Input: part model. Units: mm. Frame: model coordinates. Face numbers are marked on the shaded views. Coordinates: 2 decimals unless noted, no trailing zeros. Write each loop counter-clockwise with the first axis right and the second up, starting at its lowest first coordinate (ties: lowest second). Pieces come first, ordered by that corner, then holes. Notation, with made-up numbers: (65.5, -39) - (91.5, -39) arc R32 cw to (91.5, -3) - close; hole circle Ø3 at (18, 39). An arc over 180 degrees is marked (long way). Put each result on its own line as item: value. Start each with the question number.
1. Cut plane D-D, the plane y = 2. Return loops of the section in (x, z), and give its area (3 significant figures).
2. Pull-direction query (Z, two-part tool) for the marked faces 1, 2 and 3; classes: released by +Z, released by -Z, zero draft, split by the parting line, or undercut.
3. Cut plane B-B, the plane y = -2.5. Return loops of the section in (x, z), and give its area (3 significant figures).
4. Cut plane C-C, the plane z = 0. Return loops of the section in (x, y), and give its area (3 significant figures).
5. Cut plane A-A, the plane x = 4.5. Return loops of the section in (y, z) (3 decimals).
6. Line query: line 1 (Y direction, x = 11.25, z = 0); line 2 (Y direction, x = 4.5, z = 11.5); line 3 (Y direction, x = 2.5, z = 0.5). Output: solid intervals per line, ascending.
7. Pin query (flat end, axial travel): pin 1 (2 mm diameter, centred on y = -9, z = 2.5, fed in from -X); pin 2 (8 mm diameter, centred on x = 6.5, z = -6.5, fed in from -Y); pin 3 (3 mm diameter, centred on x = 4.5, y = -6, fed in from -Z); pin 4 (1 mm diameter, centred on x = 10, z = -0.5, fed in from +Y). Return the tip coordinate at first contact, or that it passes through.
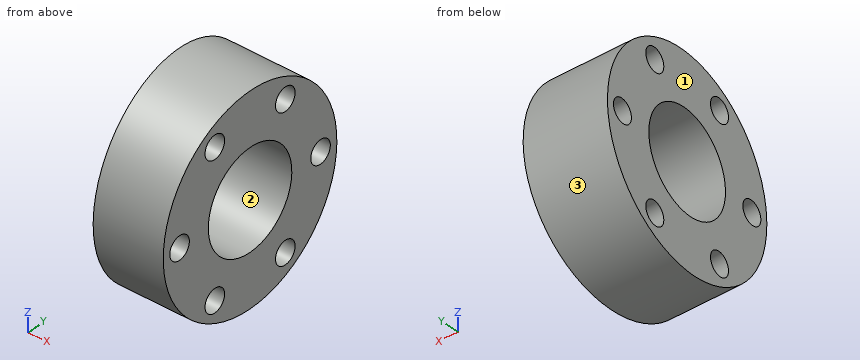
from build123d import *

# Parameters (mm, degrees)
SKETCH1_R               = 16.891
BOSS_EXTRUDE1_DEPTH     = 13.97
SKETCH2_R               = 8.128
CUT_EXTRUDE1_DEPTH      = 28.672597674
CUT_EXTRUDE2_DEPTH      = 28.672597674
CUT_EXTRUDE2_DEPTH_BACK = 28.672597674
SKETCH7_R               = 1.905
CUT_EXTRUDE3_DEPTH      = 28.672597674
CIRPATTERN1_COUNT       = 6


with BuildPart() as part:
    # Sketch1 → Boss-Extrude1 (new body)
    with BuildSketch(Plane(origin=(0, 0, 0), x_dir=(0, 0, -1), z_dir=(1, 0, 0))):
        Circle(SKETCH1_R)
    extrude(amount=BOSS_EXTRUDE1_DEPTH)

    # Sketch2 → Cut-Extrude1 (cut, through all)
    with BuildSketch(Plane(origin=(13.97, 0, 0), x_dir=(0, 0, -1), z_dir=(1, 0, 0))):
        Circle(SKETCH2_R)
    extrude(amount=-CUT_EXTRUDE1_DEPTH, mode=Mode.SUBTRACT)

    # Sketch3 → Cut-Extrude2 (cut, two sides: drawn at the far end of the back side and taken through both)
    with BuildSketch(Plane.XY.offset(-CUT_EXTRUDE2_DEPTH_BACK)):
        Polygon((0, 16.891), (2.362267561, -16.891), (0, -16.891), align=None)
    extrude(amount=CUT_EXTRUDE2_DEPTH + CUT_EXTRUDE2_DEPTH_BACK, mode=Mode.SUBTRACT)

    # Sketch7 → Cut-Extrude3 (cut, through all)
    with BuildSketch(Plane(origin=(13.97, 0, 0), x_dir=(0, 0, -1), z_dir=(1, 0, 0))):
        with Locations((0, 13.716)):
            Circle(SKETCH7_R)
    cut_extrude3 = extrude(amount=-CUT_EXTRUDE3_DEPTH, mode=Mode.SUBTRACT)

    # CirPattern1: Cut-Extrude3 ×6 about axis
    cirpattern1_axis = Axis((0, 0, 0), (1, 0, 0))
    for i in range(1, CIRPATTERN1_COUNT):
        add(cut_extrude3.rotate(cirpattern1_axis, i * 360 / CIRPATTERN1_COUNT), mode=Mode.SUBTRACT)


solid = part.part
Report:
1. outline: (1.04, -16.77) - (13.97, -16.77) - (13.97, -7.88) - (1.04, -7.88) - close; (1.04, 7.88) - (13.97, 7.88) - (13.97, 16.77) - (1.04, 16.77) - close
1. area: 230 mm^2
2. face 1: zero draft
2. face 2: undercut
2. face 3: split by the parting line
3. outline: (1.36, -16.7) - (13.97, -16.7) - (13.97, -7.73) - (1.36, -7.73) - close; (1.36, 7.73) - (13.97, 7.73) - (13.97, 16.7) - (1.36, 16.7) - close
3. area: 226 mm^2
4. outline: (0, 16.89) - (0.09, 15.62) - (13.97, 15.62) - (13.97, 16.89) - close; (0.36, 11.81) - (0.61, 8.13) - (13.97, 8.13) - (13.97, 11.81) - close; (1.75, -8.13) - (2.01, -11.81) - (13.97, -11.81) - (13.97, -8.13) - close; (2.27, -15.62) - (2.36, -16.89) - (13.97, -16.89) - (13.97, -15.62) - close
4. area: 127 mm^2
5. outline: circle Ø33.782 at (0, 0); hole circle Ø3.81 at (-13.716, 0); hole circle Ø3.81 at (-6.858, -11.878); hole circle Ø3.81 at (-6.858, 11.878); hole circle Ø16.256 at (0, 0); hole circle Ø3.81 at (6.858, -11.878); hole circle Ø3.81 at (6.858, 11.878); hole circle Ø3.81 at (13.716, 0)
6. line 1: y = -16.89 to -15.62, -11.81 to -8.13, 8.13 to 11.81, 15.62 to 16.89
6. line 2: y = -12.37 to -8.73, -4.99 to 4.99, 8.73 to 12.37
6. line 3: y = -16.88 to -15.55, -11.88 to -8.11, 8.11 to 11.88, 15.55 to 16.88
7. pin 1: stops at x = 1.74
7. pin 2: stops at y = -16.7
7. pin 3: stops at z = -16.28
7. pin 4: stops at y = 16.89
